from build123d import *

# Parameters (mm, degrees)
Y_KSEKLIK_EKSTR_ZYON1_DEPTH = 3
IZIM2_R                     = 16
KES_EKSTR_ZYON1_DEPTH       = 10
IZIM3_R                     = 1.5
KES_EKSTR_ZYON2_DEPTH       = 10
IZIM4_R                     = 4
KES_EKSTR_ZYON3_DEPTH       = 10
IZIM5_W                     = 28
IZIM5_H                     = 23
KES_EKSTR_ZYON4_DEPTH       = 10
IZIM6_W                     = 33
IZIM6_H                     = 31
KES_EKSTR_ZYON5_DEPTH       = 1.5
IZIM7_R                     = 18
IZIM7_R_2                   = 16
Y_KSEKLIK_EKSTR_ZYON2_DEPTH = 4
RADYUS1_R                   = 1
Y_KSEKLIK_EKSTR_ZYON3_START = -1.5
Y_KSEKLIK_EKSTR_ZYON3_DEPTH = 1.5
KES_EKSTR_ZYON6_DEPTH       = 4
IZIM12_W                    = 28
IZIM12_H                    = 19
KES_EKSTR_ZYON7_DEPTH       = 10
IZIM13_W                    = 33
IZIM13_H                    = 31
IZIM13_W_2                  = 28
IZIM13_H_2                  = 19
Y_KSEKLIK_EKSTR_ZYON4_DEPTH = 1.5
IZIM14_W                    = 28
IZIM14_H                    = 2.5
KES_EKSTR_ZYON8_DEPTH       = 10
IZIM15_W                    = 28
IZIM15_H                    = 2.5
Y_KSEKLIK_EKSTR_ZYON5_DEPTH = 3


with BuildPart() as part:
    # Çizim1 → Yükseklik-Ekstrüzyon1 (new body)
    with BuildSketch(Plane(origin=(0, 0, 0), x_dir=(1, 0, 0), z_dir=(0, 1, 0))):
        with BuildLine():
            Line((3.903882032, 0), (112.096117968, 0))
            ThreePointArc((112.096117968, 0), (115.173179015, -1.05897281), (116.946830469, -3.787321875))
            Line((116.946830469, -3.787321875), (136.446830469, -81.787321875))
            ThreePointArc((136.446830469, -81.787321875), (135.537145158, -86.077061047), (131.596117968, -88))
            Line((131.596117968, -88), (96.903882032, -88))
            ThreePointArc((96.903882032, -88), (93.826820985, -86.94102719), (92.053169531, -84.212678125))
            Line((92.053169531, -84.212678125), (90.946830469, -79.787321875))
            ThreePointArc((90.946830469, -79.787321875), (89.173179015, -77.05897281), (86.096117968, -76))
            Line((86.096117968, -76), (29.903882032, -76))
            ThreePointArc((29.903882032, -76), (26.826820985, -77.05897281), (25.053169531, -79.787321875))
            Line((25.053169531, -79.787321875), (23.946830469, -84.212678125))
            ThreePointArc((23.946830469, -84.212678125), (22.173179015, -86.94102719), (19.096117968, -88))
            Line((19.096117968, -88), (-15.596117968, -88))
            ThreePointArc((-15.596117968, -88), (-19.537145158, -86.077061047), (-20.446830469, -81.787321875))
            Line((-20.446830469, -81.787321875), (-0.946830469, -3.787321875))
            ThreePointArc((-0.946830469, -3.787321875), (0.826820985, -1.05897281), (3.903882032, 0))
        make_face()
    extrude(amount=Y_KSEKLIK_EKSTR_ZYON1_DEPTH)

    # Çizim2 → Kes-Ekstrüzyon1 (cut)
    with BuildSketch(Plane(origin=(0, 3, 0), x_dir=(1, 0, 0), z_dir=(0, 1, 0))):
        with Locations(Location((16.91, -45.35, 0), (0, 0, 270))):
            Circle(IZIM2_R)
        with Locations(Location((97.41, -45.35, 0), (0, 0, 270))):
            Circle(IZIM2_R)
    extrude(amount=-KES_EKSTR_ZYON1_DEPTH, mode=Mode.SUBTRACT)

    # Çizim3 → Kes-Ekstrüzyon2 (cut)
    with BuildSketch(Plane(origin=(0, 3, 0), x_dir=(1, 0, 0), z_dir=(0, 1, 0))):
        with Locations(Location((5.6, -7.73, 0), (0, 0, 270))):
            Circle(IZIM3_R)
        with Locations(Location((-11.94, -80.5, 0), (0, 0, 270))):
            Circle(IZIM3_R)
        with Locations(Location((127.94, -80.5, 0), (0, 0, 90))):
            Circle(IZIM3_R)
        with Locations(Location((110.4, -7.73, 0), (0, 0, 90))):
            Circle(IZIM3_R)
    extrude(amount=-KES_EKSTR_ZYON2_DEPTH, mode=Mode.SUBTRACT)

    # Çizim4 → Kes-Ekstrüzyon3 (cut)
    with BuildSketch(Plane(origin=(0, 3, 0), x_dir=(1, 0, 0), z_dir=(0, 1, 0))):
        with Locations(Location((38.16, -23.5, 0), (0, 0, 270))):
            Circle(IZIM4_R)
        with Locations(Location((57.16, -23.5, 0), (0, 0, 270))):
            Circle(IZIM4_R)
        with Locations(Location((77.16, -23.5, 0), (0, 0, 270))):
            Circle(IZIM4_R)
    extrude(amount=-KES_EKSTR_ZYON3_DEPTH, mode=Mode.SUBTRACT)

    # Çizim5 → Kes-Ekstrüzyon4 (cut)
    with BuildSketch(Plane(origin=(0, 3, 0), x_dir=(1, 0, 0), z_dir=(0, 1, 0))):
        with Locations((57.16, -52.3)):
            Rectangle(IZIM5_W, IZIM5_H)
    extrude(amount=-KES_EKSTR_ZYON4_DEPTH, mode=Mode.SUBTRACT)

    # Çizim6 → Kes-Ekstrüzyon5 (cut)
    with BuildSketch(Plane(origin=(0, 3, 0), x_dir=(1, 0, 0), z_dir=(0, 1, 0))):
        with Locations((57.16, -52.3)):
            Rectangle(IZIM6_W, IZIM6_H)
    extrude(amount=-KES_EKSTR_ZYON5_DEPTH, mode=Mode.SUBTRACT)

    # Çizim7 → Yükseklik-Ekstrüzyon2 (add)
    # profile 1 of 2: a face of its own
    with BuildSketch(Plane.XZ):
        with Locations(Location((97.41, 45.35, 0), (0, 0, 270))):
            Circle(IZIM7_R)
        with Locations(Location((97.41, 45.35, 0), (0, 0, 90))):
            Circle(IZIM7_R_2, mode=Mode.SUBTRACT)
    # profile 2 of 2: a face of its own
    with BuildSketch(Plane.XZ):
        with Locations(Location((16.91, 45.35, 0), (0, 0, 270))):
            Circle(IZIM7_R)
        with Locations(Location((16.91, 45.35, 0), (0, 0, 90))):
            Circle(IZIM7_R_2, mode=Mode.SUBTRACT)
    extrude(amount=Y_KSEKLIK_EKSTR_ZYON2_DEPTH)

    # Çizim8 → Döndür1 (revolve)
    with BuildSketch(Plane.XY.offset(45.35), mode=Mode.PRIVATE) as d_nd_r1_sk:
        with BuildLine():
            Line((112.41, -5.015624143), (112.41, -7))
            ThreePointArc((112.41, -7), (114.070930331, -5.660930331), (115.41, -4))
            Line((115.41, -4), (113.425624143, -4))
            ThreePointArc((113.425624143, -4), (112.939559481, -4.529559481), (112.41, -5.015624143))
        make_face()
    revolve(d_nd_r1_sk.sketch.rotate(Axis((97.41, -4, 45.35), (0, -1, 0)), 90), axis=Axis((97.41, -4, 45.35), (0, -1, 0)))

    # Çizim9 → Döndür2 (revolve)
    with BuildSketch(Plane.XY.offset(45.35), mode=Mode.PRIVATE) as d_nd_r2_sk:
        with BuildLine():
            Line((31.91, -5.473337822), (31.91, -7))
            ThreePointArc((31.91, -7), (33.570930331, -5.660930331), (34.91, -4))
            Line((34.91, -4), (33.383337822, -4))
            ThreePointArc((33.383337822, -4), (32.690654868, -4.780654868), (31.91, -5.473337822))
        make_face()
    revolve(d_nd_r2_sk.sketch.rotate(Axis((16.91, -4, 45.35), (0, -1, 0)), 180), axis=Axis((16.91, -4, 45.35), (0, -1, 0)))

    # Radyus1
    radyus1_edges = [part.edges().sort_by_distance(p)[0] for p in [
        (97.41, 0, 63.35),
        (16.91, 0, 63.35),
    ]]
    fillet(radyus1_edges, radius=RADYUS1_R)

    # Çizim10 → Yükseklik-Ekstrüzyon3 (add)
    with BuildSketch(Plane(origin=(0, 0, 0), x_dir=(-1, 0, 0), z_dir=(0, -1, 0)).offset(Y_KSEKLIK_EKSTR_ZYON3_START)):
        Polygon((-70.36, -40.8), (-70.36, -56.3), (-43.16, -56.3), (-43.16, -63.8), (-71.16, -63.8), (-71.16, -40.8), align=None)
    extrude(amount=Y_KSEKLIK_EKSTR_ZYON3_DEPTH)

    # Çizim11 → Kes-Ekstrüzyon6 (cut)
    with BuildSketch(Plane.XZ):
        Polygon((42.86, 40.5), (42.86, 56.3), (43.16, 56.3), (43.16, 40.8), (70.36, 40.8), (70.36, 40.5), align=None)
    extrude(amount=-KES_EKSTR_ZYON6_DEPTH, mode=Mode.SUBTRACT)

    # Çizim12 → Kes-Ekstrüzyon7 (cut)
    with BuildSketch(Plane(origin=(0, 1.5, 0), x_dir=(1, 0, 0), z_dir=(0, 1, 0))):
        with Locations((56.86, -48.4)):
            Rectangle(IZIM12_W, IZIM12_H)
    extrude(amount=-KES_EKSTR_ZYON7_DEPTH, mode=Mode.SUBTRACT)

    # Çizim13 → Yükseklik-Ekstrüzyon4 (add)
    with BuildSketch(Plane(origin=(0, 1.5, 0), x_dir=(1, 0, 0), z_dir=(0, 1, 0))):
        with Locations((57.16, -52.3)):
            Rectangle(IZIM13_W, IZIM13_H)
        with Locations((56.86, -48.4)):
            Rectangle(IZIM13_W_2, IZIM13_H_2, mode=Mode.SUBTRACT)
    extrude(amount=Y_KSEKLIK_EKSTR_ZYON4_DEPTH)

    # Çizim14 → Kes-Ekstrüzyon8 (cut)
    with BuildSketch(Plane(origin=(0, 3, 0), x_dir=(1, 0, 0), z_dir=(0, 1, 0))):
        with Locations((56.86, -59.15)):
            Rectangle(IZIM14_W, IZIM14_H)
    extrude(amount=-KES_EKSTR_ZYON8_DEPTH, mode=Mode.SUBTRACT)

    # Çizim15 → Yükseklik-Ekstrüzyon5 (add)
    with BuildSketch(Plane(origin=(0, 3, 0), x_dir=(1, 0, 0), z_dir=(0, 1, 0))):
        with Locations((56.86, -40.15)):
            Rectangle(IZIM15_W, IZIM15_H)
    extrude(amount=-Y_KSEKLIK_EKSTR_ZYON5_DEPTH)


solid = part.part
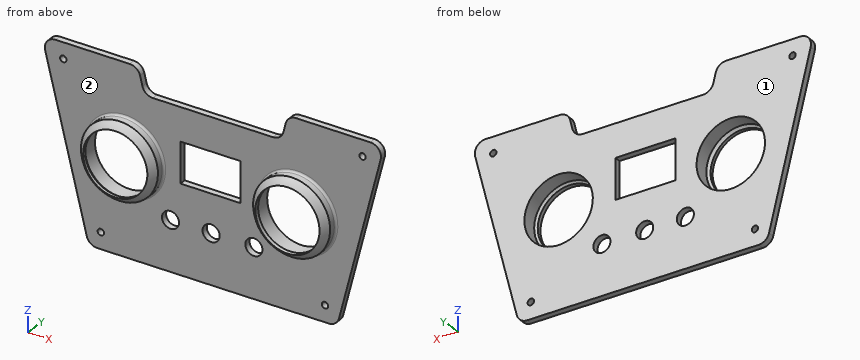
For this review, take the finished solid that the model builds, in its own axes (mm). Face numbers are marked on the shaded views. Round coordinates to 2 decimals unless told otherwise and drop trailing zeros. Loops run counter-clockwise (first coordinate to the right, second up) from the corner with the lowest first, then second, coordinate; pieces in that order, holes last. Notation, with made-up numbers: (-35.75, 4) - (-10.75, 4) arc R31 ccw to (-10.75, 41) - close; hole circle Ø9 at (85.5, 16.25). An arc over 180 degrees is marked (long way). Answer as CSV lines item,"result".
(1) Wall thickness on line 1 (X direction, y = -3.75, z = 46); line 2 (Z direction, x = 17, y = -2); line 3 (X direction, y = 1.3, z = 7.73): over which ranges is each line inside the solid? List them lowest first.
Checked values:
line 1,"x = -1.08 to 0.92, 32.9 to 34.9, 79.42 to 81.42, 113.4 to 115.4"
line 2,"z = 27.35 to 29.35, 61.35 to 63.35"
line 3,"x = -1.93 to 4.1, 7.1 to 108.9, 111.9 to 117.93"
(2) Mouldability with a two-part tool opening along X and no side actions: class the marked faces 1 and 2 as +X half, -X half, draft (parallel to the pull), parting line (faces both ways), or undercut.
Checked values:
face 1,"draft"
face 2,"undercut"
(3) Consider section A-A on x = 127.94. Give the boundary of the cut face in (y, z), then the cut area to 3 significant figures.
Checked values:
outline,"(0, 47.76) - (3, 47.76) - (3, 79) - (0, 79) - close; (0, 82) - (3, 82) - (3, 88) - (0, 88) - close"
area,"112 mm2"
(4) Insertion check: P1, Ø7, axis at x = 57.16, z = 23.5, coming from the -Y side; P2, Ø1.5, axis at y = 2, z = 48, coming from the +X side; P3, Ø1.5, axis at y = -3.5, z = 40.5, coming from the +X side; P4, Ø0.9, axis at x = 60.5, y = 1, coming from the +Z side. Each pin has a flat end and moves straight along its axis. Give the tip position at first contact, or say it passes through.
Checked values:
P1,"passes through"
P2,"stops at x = 128.19"
P3,"stops at x = 114.94"
P4,"stops at z = 76"
(5) Consider section B-B on x = 57.16. Give the boundary of the cut face in (y, z).
Checked values:
outline,"(0, 0) - (3, 0) - (3, 19.5) - (0, 19.5) - close; (0, 27.5) - (3, 27.5) - (3, 41.4) - (0, 41.4) - close; (0, 60.4) - (3, 60.4) - (3, 76) - (0, 76) - close"
(6) Consider section C-C on z = 23.5. Give the boundary of the cut face in (x, y) (3 decimals), then the cut area to 3 significant figures.
Checked values:
outline,"(-5.875, 0) - (34.16, 0) - (34.16, 3) - (-5.875, 3) - close; (42.16, 0) - (53.16, 0) - (53.16, 3) - (42.16, 3) - close; (61.16, 0) - (73.16, 0) - (73.16, 3) - (61.16, 3) - close; (81.16, 0) - (121.875, 0) - (121.875, 3) - (81.16, 3) - close"
area,"311 mm2"
(7) Consider section D-D on z = 72. Give the boundary of the cut face in (x, y), then the cut area to 3 significant figures.
Checked values:
outline,"(-18, 0) - (134, 0) - (134, 3) - (-18, 3) - close"
area,"456 mm2"
